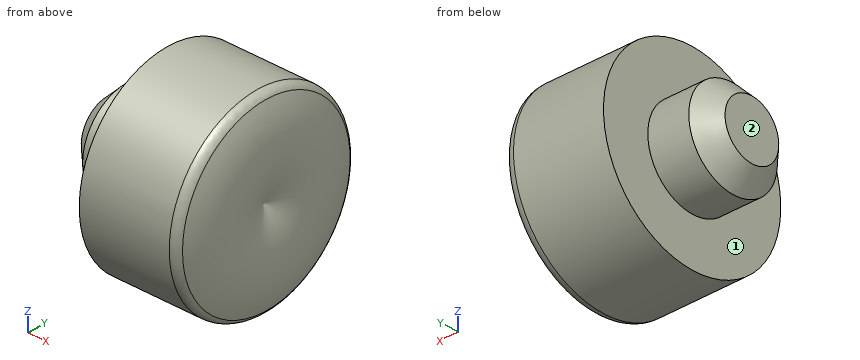
from build123d import *

# Parameters (mm, degrees)
F2_SIZE  = 1
F3_R     = 0.5
F6_DEPTH = 3.4


with BuildPart() as f1:
    # F0 (on Front) → F1 (revolve)
    with BuildSketch(Plane.XZ):
        with BuildLine():
            Line((0, 5.08), (0, 2.54))
            Line((0, 2.54), (-3.175, 2.54))
            Line((-3.175, 2.54), (-3.175, 0))
            Line((-3.175, 0), (5.08, 0))
            ThreePointArc((5.08, 0), (5.760591, 2.54), (5.08, 5.08))
            Line((5.08, 5.08), (0, 5.08))
        make_face()
    revolve(axis=Axis((-24.371815, 0, 0), (-1, 0, 0)))

    # F2
    f2_edges = [f1.edges().sort_by_distance(p)[0] for p in [
        (-3.175, 0, -2.54),
    ]]
    chamfer(f2_edges, length=F2_SIZE)

    # F3
    f3_edges = [f1.edges().sort_by_distance(p)[0] for p in [
        (5.08, 0, -5.08),
    ]]
    fillet(f3_edges, radius=F3_R)

    # F5 (on offset) → F6 (cut)
    with BuildSketch(Plane.YZ.offset(4.5)):
        Polygon((0, -3.117691), (2.7, -1.558846), (2.7, 1.558846), (0, 3.117691), (-2.7, 1.558846), (-2.7, -1.558846), align=None)
    extrude(amount=-F6_DEPTH, mode=Mode.SUBTRACT)


solid = f1.part
CAD build for the part. Positions are in the model's coordinates, mm. Face numbers are marked on the shaded views. A direction names the side the tool comes from. Round coordinates to 2 decimals unless told otherwise and drop trailing zeros. Write each loop counter-clockwise with the first axis right and the second up, starting at its lowest first coordinate (ties: lowest second). Pieces come first, ordered by that corner, then holes. Notation, with made-up numbers: M 68.25,-3 L 86.25,-3 A4 cw 86.25,1 Z; hole C 4.25,-19 d5. An arc over 180 degrees is marked long. Put each result on its own line as item: value. Start each with the question number.
1) 3-axis set-ups, long thin cutter, end or side, ignore diameter. For the marked faces 1 and 2: which of +Z, -Z, +X, -X, +Y, -Y reach the whole face in a straight line?
2) Drill centre lines: probe 1 along X at (y, z) = (-3, 3.75); probe 2 along X at (y, z) = (-1.5, 0.25) (3 decimals); probe 3 along X at (y, z) = (-1.5, -1). Where is each one in solid material? Low to high. Write a range as [from, to].
3) Saw through at A-A, the plane x = 1.5. Write the cut outline in (y, z).
4) Pin check, flat tips, straight feed: pin 1 Ø1.6 at (y, z) = (0.5, 0.5) entering from +X; pin 2 Ø5 at (x, y) = (-1.5, -2.5) entering from -Z; pin 3 Ø1.5 at (y, z) = (0.5, 2.5) entering from -X. Stop position of each tip, or through.
5) Saw through at C-C, the plane x = -2.5. Write the cut outline in (y, z) (3 decimals), and give its area (3 significant figures).
6) Saw through at B-B, the plane x = -0.75. Write the cut outline in (y, z), and give its area (3 significant figures).
Resolved:
1. face 1: -X
1. face 2: +Z, -Z, -X, +Y, -Y
2. probe 1: [0, 5.23]
2. probe 2: [-3.175, 1.1], [4.5, 5.657]
2. probe 3: [-2.91, 1.1], [4.5, 5.71]
3. outline: C 0,0 d10.16; hole M -2.7,-1.56 L 0,-3.12 L 2.7,-1.56 L 2.7,1.56 L 0,3.12 L -2.7,1.56 Z
4. pin 1: x = 5.65
4. pin 2: z = -5.06
4. pin 3: x = -2.92
5. outline: C 0,0 d4.43
5. area: 15.4 mm²
6. outline: C 0,0 d5.08
6. area: 20.3 mm²
